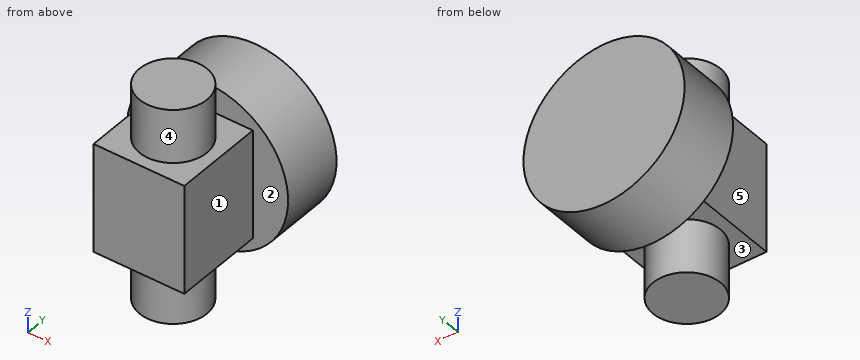
from build123d import *

# Parameters (mm, degrees)
SKETCH1_W           = 19.05
SKETCH1_H           = 22.86
BOSS_EXTRUDE1_DEPTH = 9.525
SKETCH2_R           = 16.92275
BOSS_EXTRUDE2_DEPTH = 13.462
SKETCH4_R           = 7.08025
BOSS_EXTRUDE4_DEPTH = 22.6695


with BuildPart() as part:
    # Sketch1 → Boss-Extrude1 (new, symmetric)
    with BuildSketch(Plane(origin=(0, 0, 0), x_dir=(1, 0, 0), z_dir=(0, 1, 0))):
        Rectangle(SKETCH1_W, SKETCH1_H)
    extrude(amount=BOSS_EXTRUDE1_DEPTH, both=True)

    # Sketch2 → Boss-Extrude2 (add)
    with BuildSketch(Plane(origin=(0, 9.525, 0), x_dir=(1, 0, 0), z_dir=(0, 1, 0))):
        with Locations(Location((0, 0, 0), (0, 0, 270))):
            Circle(SKETCH2_R)
    extrude(amount=BOSS_EXTRUDE2_DEPTH)

    # Sketch4 → Boss-Extrude4 (add, symmetric)
    with BuildSketch(Plane.XY):
        with Locations(Location((0, 0, 0), (0, 0, 180))):
            Circle(SKETCH4_R)
    extrude(amount=BOSS_EXTRUDE4_DEPTH, both=True)


solid = part.part
For this review, take the finished solid that the model builds, in its own axes (mm). Face numbers are marked on the shaded views. A direction names the side the tool comes from. Coordinates: 2 decimals unless noted, no trailing zeros. Write each loop counter-clockwise with the first axis right and the second up, starting at its lowest first coordinate (ties: lowest second). Pieces come first, ordered by that corner, then holes. Notation, with made-up numbers: (72.5, -1.5) -> (79.5, -1.5) arc R19 ccw to (79.5, 9.5) -> close; hole circle Ø1 at (70, 14.25). An arc over 180 degrees is marked (long way). Write each question's results on one line, items separated by ' | '. Start each with the question number.
1) Consider section D-D (z = 0). Write out the cut boundary in (x, y) (3 decimals).
2) For the marked faces 1, 2, 3, 4 and 5, list the 3-axis set-ups (+Z, -Z, +X, -X, +Y, -Y) from which the entire face can be reached by the end or side of a thin tool; tool diameter is ignored.
3) Consider section B-B (y = 2.5). Write out the cut boundary in (x, z) (1 decimal), plus the area to 3 significant figures.
4) Insertion check: pin 1 (1 mm diameter, centred on y = 2, z = 4.5, fed in from +X) (3 decimals); pin 2 (3 mm diameter, centred on y = 16.5, z = 16.5, fed in from -X); pin 3 (5.5 mm diameter, centred on y = 3, z = -5, fed in from -X) (3 decimals). Each pin has a flat end and moves straight along its axis. Give the tip position at first contact, or say it passes through.
5) Wall thickness on L1, parallel to Y at x = -5.5, z = -13.5 (3 decimals); L2, parallel to X at y = -6.5, z = 3.5 (3 decimals); L3, parallel to Y at x = -10, z = 9 (3 decimals): over which ranges is each line inside the solid? List them lowest first. Write a range as [from, to].
6) Consider section C-C (x = 0). Write out the cut boundary in (y, z) (1 decimal).
7) Consider section A-A (z = 13.5). Write out the cut boundary in (x, y) (1 decimal), plus the area to 3 significant figures.
Geometry says:
1) outline: (-16.923, 9.525) -> (-9.525, 9.525) -> (-9.525, -9.525) -> (9.525, -9.525) -> (9.525, 9.525) -> (16.923, 9.525) -> (16.923, 22.987) -> (-16.923, 22.987) -> close
2) face 1: +Z, -Z, +X, -Y | face 2: none | face 3: -Z | face 4: +Z | face 5: +Z, -Z, -X, -Y
3) outline: (-9.5, -11.4) -> (-6.6, -11.4) -> (-6.6, -22.7) -> (6.6, -22.7) -> (6.6, -11.4) -> (9.5, -11.4) -> (9.5, 11.4) -> (6.6, 11.4) -> (6.6, 22.7) -> (-6.6, 22.7) -> (-6.6, 11.4) -> (-9.5, 11.4) -> close | area: 733 mm^2
4) pin 1: x = 9.525 | pin 2: x = -7.83 | pin 3: x = -9.525
5) L1: [-4.459, 4.459], [9.525, 22.987] | L2: [-9.525, 9.525] | L3: [9.525, 22.987]
6) outline: (-9.5, -11.4) -> (-7.1, -11.4) -> (-7.1, -22.7) -> (7.1, -22.7) -> (7.1, -11.4) -> (9.5, -11.4) -> (9.5, -16.9) -> (23, -16.9) -> (23, 16.9) -> (9.5, 16.9) -> (9.5, 11.4) -> (7.1, 11.4) -> (7.1, 22.7) -> (-7.1, 22.7) -> (-7.1, 11.4) -> (-9.5, 11.4) -> close
7) outline: (-10.2, 9.5) -> (10.2, 9.5) -> (10.2, 23) -> (-10.2, 23) -> close; circle Ø14.2 at (0, 0) | area: 432 mm^2
